```python
from build123d import *

# Parameters (mm, degrees)
F0_W     = 33.02
F0_H     = 38.1
F1_DEPTH = 3.81
F2_R     = 25.20878
F2_R_2   = 20.12878
F3_DEPTH = 25.4
F4_R     = 14.732
F5_DEPTH = 25.4


with BuildPart() as f1:
    # F0 (on Front) → F1 (new body)
    with BuildSketch(Plane.XZ):
        Rectangle(F0_W, F0_H)
    extrude(amount=F1_DEPTH)

    # F2 (on face) → F3 (cut)
    with BuildSketch(Plane.XZ.offset(3.81)):
        Circle(F2_R)
        Circle(F2_R_2, mode=Mode.SUBTRACT)
    extrude(amount=-F3_DEPTH, mode=Mode.SUBTRACT)

    # F4 (on face) → F5 (cut)
    with BuildSketch(Plane.XZ.offset(3.81)):
        Circle(F4_R)
    extrude(amount=-F5_DEPTH, mode=Mode.SUBTRACT)


solid = f1.part
```
Geometry check sheet. Reference: the model listing, model coordinates, mm. Give positions to 0.01 mm unless a question says otherwise; leave off trailing zeros. Write each loop counter-clockwise with the first axis right and the second up, starting at its lowest first coordinate (ties: lowest second). Pieces come first, ordered by that corner, then holes. Notation, with made-up numbers: (-27, 18.25) -> (-2, 18.25) arc R23 cw to (-2, 40.25) -> close; hole circle Ø5 at (72.5, 31.5). An arc over 180 degrees is marked (long way). Use one line per item in the form item = value.
Item 1: Sectioned sample at A-A on z = 0. Enter the section's corners in (x, y).
Results list:
outline = (-16.51, -3.81) -> (-14.73, -3.81) -> (-14.73, 0) -> (-16.51, 0) -> close; (14.73, -3.81) -> (16.51, -3.81) -> (16.51, 0) -> (14.73, 0) -> close
Item 2: Depth check by flat-ended pin: pin 1 Ø8 at (x, z) = (6.5, 2) entering from -Y; pin 2 Ø1 at (x, y) = (8, -1.5) entering from +Z. Enter the tip coordinate at first touch or a pass-through.
Results list:
pin_1 = through
pin_2 = 18.68
Item 3: Sectioned sample at B-B on x = 14. Enter the section's corners in (y, z), plus the area to 3 significant figures.
Results list:
outline = (-3.81, -14.46) -> (0, -14.46) -> (0, -4.59) -> (-3.81, -4.59) -> close; (-3.81, 4.59) -> (0, 4.59) -> (0, 14.46) -> (-3.81, 14.46) -> close
area = 75.3 mm2
Item 4: Sectioned sample at C-C on y = -3. Enter the section's corners in (x, z).
Results list:
outline = (-16.51, -11.51) arc R20.13 ccw to (-6.5, -19.05) -> (6.5, -19.05) arc R20.13 ccw to (16.51, -11.51) -> (16.51, 11.51) arc R20.13 ccw to (6.5, 19.05) -> (-6.5, 19.05) arc R20.13 ccw to (-16.51, 11.51) -> close; hole circle Ø29.46 at (0, 0)
Item 5: Scan lines: line 1 (Z direction, x = 0, y = -2.85); line 2 (X direction, y = -2.8, z = -13). Record each from-to range of solid material in increasing order.
Results list:
line_1 = -19.05 to -14.73, 14.73 to 19.05
line_2 = -15.37 to -6.93, 6.93 to 15.37
